```python
from build123d import *

# Parameters (mm, degrees)
F0_R     = 6
F1_DEPTH = 200
F3_R     = 5
F4_DEPTH = 10
F5_DEPTH = 210


with BuildPart() as f1:
    # F0 (on Top) → F1 (new body)
    with BuildSketch(Plane.XY):
        Circle(F0_R)
    extrude(amount=F1_DEPTH)

    # F3 (on face) → F4 (join)
    with BuildSketch(Plane.XY.offset(200)):
        Circle(F3_R)
    extrude(amount=F4_DEPTH)

    # F3 (on face) → F5 (join)
    with BuildSketch(Plane.XY.offset(200)):
        Circle(F3_R)
    extrude(amount=-F5_DEPTH)


solid = f1.part
```
For this review, take the finished solid that the model builds, in its own axes (mm). A direction names the side the tool comes from. Round coordinates to 2 decimals unless told otherwise and drop trailing zeros. Write each loop counter-clockwise with the first axis right and the second up, starting at its lowest first coordinate (ties: lowest second). Pieces come first, ordered by that corner, then holes. Notation, with made-up numbers: (-21, 84.25) -> (9, 84.25) arc R30 ccw to (9, 114.25) -> close; hole circle Ø6 at (-5, 72). An arc over 180 degrees is marked (long way). One line per question, with ' | ' between items. Start each with the question number.
(1) Tool access review of faces 1 (the face through (-6, 0, 99)), 2 (the face through (-4, 4, 0)), 3 (the face through (-1.08, -4.88, 204.93)): name each direction out of +Z, -Z, +X, -X, +Y, -Y from which nothing blocks a thin tool from reaching the whole face with its end or side.
(2) Insertion check: P1, Ø1.5, axis at x = 3.5, z = 90, coming from the +Y side; P2, Ø1.5, axis at x = 4.5, z = 108.5, coming from the +Y side; P3, Ø1.5, axis at x = -4, y = 5, coming from the +Z side. Each pin has a flat end and moves straight along its axis. Give the tip position at first contact, or say it passes through.
(3) Add section C-C, the plane z = 4.5. Write out the cut boundary in (x, y), plus the area to 3 significant figures.
(4) Add section B-B, the plane x = -0.5. Write out the cut boundary in (y, z).
(5) For line 1 along Y through (x, z) = (-0.25, 106); line 2 along Z through (x, y) = (-4.5, 3); line 3 along X through (y, z) = (0.5, 49.5), list the stretches that pass through material, from the lowest coordinate up. Write a range as from..to.
(6) Add section A-A, the plane y = 0. Write out the cut boundary in (x, z).
Answer list:
1) face 1: +Z, -Z | face 2: -Z | face 3: +Z
2) P1: y = 5.33 | P2: y = 4.68 | P3: z = 200
3) outline: circle Ø12 at (0, 0) | area: 113 mm²
4) outline: (-5.98, 0) -> (-4.97, 0) -> (-4.97, -10) -> (4.97, -10) -> (4.97, 0) -> (5.98, 0) -> (5.98, 200) -> (4.97, 200) -> (4.97, 210) -> (-4.97, 210) -> (-4.97, 200) -> (-5.98, 200) -> close
5) line 1: -5.99..5.99 | line 2: 0..200 | line 3: -5.98..5.98
6) outline: (-6, 0) -> (-5, 0) -> (-5, -10) -> (5, -10) -> (5, 0) -> (6, 0) -> (6, 200) -> (5, 200) -> (5, 210) -> (-5, 210) -> (-5, 200) -> (-6, 200) -> close
